Could you check a few things on this drawing? It's one solid part, dimensions in mm from its lowest x, y, z. A direction names the side the tool comes from. Give positions to 0.01 mm unless a question says otherwise; leave off trailing zeros. Loops run counter-clockwise (first coordinate to the right, second up) from the corner with the lowest first, then second, coordinate; pieces in that order, holes last. Notation, with made-up numbers: (-33, -37) - (-20, -37) arc R26 ccw to (-20, -21) - close; hole circle Ø7 at (41, -35.5). An arc over 180 degrees is marked (long way). Answer as a JSON object with one key per item and string values.
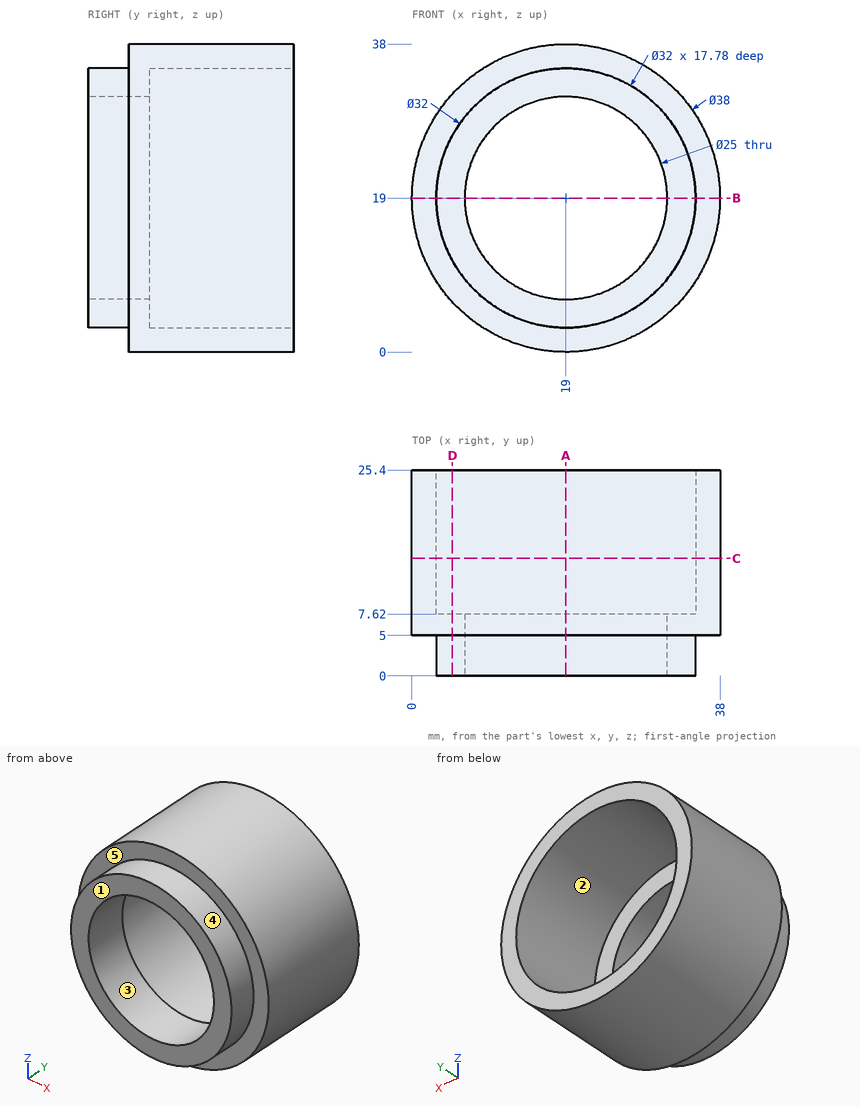
1) Imagine slicing it at B-B on z = 19. Write out the boundary of the cut face in (x, y), and give its area (3 significant figures).
Check sheet entries:
{"outline": "(0, 5) - (3, 5) - (3, 0) - (6.5, 0) - (6.5, 7.62) - (3, 7.62) - (3, 25.4) - (0, 25.4) - close; (31.5, 0) - (35, 0) - (35, 5) - (38, 5) - (38, 25.4) - (35, 25.4) - (35, 7.62) - (31.5, 7.62) - close", "area": "176 mm2"}
2) Imagine slicing it at A-A on x = 19. Write out the boundary of the cut face in (y, z), and give its area (3 significant figures).
Check sheet entries:
{"outline": "(0, 3) - (5, 3) - (5, 0) - (25.4, 0) - (25.4, 3) - (7.62, 3) - (7.62, 6.5) - (0, 6.5) - close; (0, 31.5) - (7.62, 31.5) - (7.62, 35) - (25.4, 35) - (25.4, 38) - (5, 38) - (5, 35) - (0, 35) - close", "area": "176 mm2"}
3) Imagine slicing it at C-C on y = 14.5. Write out the boundary of the cut face in (x, z), and give its area (3 significant figures).
Check sheet entries:
{"outline": "circle Ø38 at (19, 19); hole circle Ø32 at (19, 19)", "area": "330 mm2"}
4) I need wall thicknesses on L1, parallel to Z at x = 19, y = 13.5; L2, parallel to Y at x = 15, z = 2.5; L3, parallel to Z at x = 19, y = 4.5. Which ranges of each line are inside material? Lowest first, please.
Check sheet entries:
{"L1": "0 to 3, 35 to 38", "L2": "5 to 25.4", "L3": "3 to 6.5, 31.5 to 35"}
5) Which directions (+Z, -Z, +X, -X, +Y, -Y) give clear straight access to the entire face, cutting with the end or side of a thin tool? Please do the marked faces 1 and 2.
Check sheet entries:
{"face 1": "+Z, -Z, +X, -X, -Y", "face 2": "+Y"}
6) If we mould it in two halves opening along X, with no side actions, what happens to the marked faces 3, 4 and 5? For each: released by +X, released by -X, zero draft, split by the parting line, or undercut.
Check sheet entries:
{"face 3": "undercut", "face 4": "split by the parting line", "face 5": "zero draft"}
7) Imagine slicing it at D-D on x = 5. Write out the boundary of the cut face in (y, z).
Check sheet entries:
{"outline": "(0, 11.25) - (5, 11.25) - (5, 6.15) - (25.4, 6.15) - (25.4, 11.25) - (7.62, 11.25) - (7.62, 26.75) - (25.4, 26.75) - (25.4, 31.85) - (5, 31.85) - (5, 26.75) - (0, 26.75) - close"}
8) I'm going to push flat-ended pins straight in: P1, Ø10, axis at x = 30, y = 11, coming from the -Z side; P2, Ø6, axis at x = 26, y = 8, coming from the -Z side; P3, Ø9.5, axis at x = 24.5, z = 11.5, coming from the +Y side; P4, Ø15, axis at x = 19, z = 19, coming from the +Y side. Where does each tip first touch, or does it pass through?
Check sheet entries:
{"P1": "z = 0.97", "P2": "z = 0.43", "P3": "y = 7.62", "P4": "through"}
